Autodesk Inventor part; units mm, degrees
ref_plane "YZ Plane" through (0, 0, 0) normal (1, 0, 0) x (0, 1, 0)
ref_plane "XZ Plane" through (0, 0, 0) normal (0, 1, 0) x (-1, 0, 0)
ref_plane "XY Plane" through (0, 0, 0) normal (0, 0, 1) x (1, 0, 0)
sketch "Sketch1" plane through (0, 0, 0) normal (0, 0, 1) x (1, 0, 0)
  line L0 (-25, -13) -> (25, -13)
  line L1 (25, -13) -> (25, 13)
  line L2 (25, 13) -> (-25, 13)
  line L3 (-25, 13) -> (-25, -13)
  line L4 (-25, -13) -> (25, 13) construction
  line L5 (25, -13) -> (-25, 13) construction
  point P0 (0, 0)
  dimension "d0" = 50
  dimension "d1" = 26
extrude "Extrusion1" add sketch "Sketch1" along normal blind 1.6
sketch "Sketch2" plane through (0, 0, 1.6) normal (0, 0, 1) x (1, 0, 0)
  line L0 (-10.2, -7.5) -> (2.8, -7.5) construction
  line L1 (2.8, -7.5) -> (2.8, 7.5) construction
  line L2 (2.8, 7.5) -> (-10.2, 7.5) construction
  line L3 (-10.2, 7.5) -> (-10.2, -7.5) construction
  line L4 (-25, 13) -> (-25, -13) construction
  point P0 (0, 0)
  point P1 (2.8, 0)
  dimension "d4" = 13
  dimension "d5" = 15
  dimension "d6" = 14.8
hole "Hole1" at (-10.2, 7.5, 1.6) at (2.8, 7.5, 1.6) at (2.8, -7.5, 1.6) at (-10.2, -7.5, 1.6) direction (0, 0, -1) diameter 4.5 end through all
sketch "Sketch3" plane through (25, -13, 0) normal (1, 0, 0) x (0, 0, -1)
  line L0 (0, 10.5) -> (-6.5, 10.5)
  line L1 (-6.5, 10.5) -> (-6.5, 15.5)
  line L2 (-6.5, 15.5) -> (0, 15.5)
  line L3 (0, 15.5) -> (0, 10.5)
  line L4 (0, 0) -> (0, 26)
  point P0 (0, 13)
  point P1 (0, 13)
  point P2 (0, 13)
  point P3 (0, 13)
  dimension "d14" = 5
  dimension "d15" = 6.5
extrude "Extrusion2" add sketch "Sketch3" along normal mid plane 16
properties part number "IGBT_Platine"
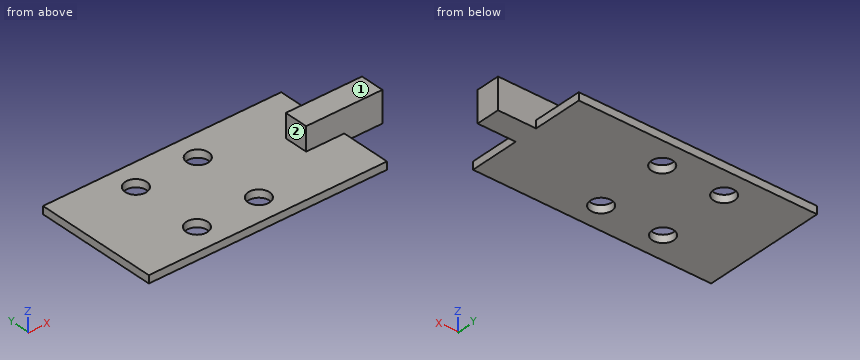
Check sheet for the modelled part. Datum: model origin and axes. Units: mm. Face numbers are marked on the shaded views. A direction names the side the tool comes from. Round coordinates to 2 decimals unless told otherwise and drop trailing zeros. Loops run counter-clockwise (first coordinate to the right, second up) from the corner with the lowest first, then second, coordinate; pieces in that order, holes last. Notation, with made-up numbers: (21.25, 4.25) -> (69.25, 4.25) arc R31 ccw to (69.25, 37.25) -> close; hole circle Ø6 at (-31.5, 4). An arc over 180 degrees is marked (long way). Write item = value, one per line. Start each with the question number.
1) Sectioned sample at C-C, the plane x = 19.5. Record the cut outline in (y, z), plus the area to 3 significant figures.
2) Sectioned sample at B-B, the plane x = -10.2. Record the cut outline in (y, z), plus the area to 3 significant figures.
3) Sectioned sample at D-D, the plane z = 5.25. Record the cut outline in (x, y).
4) Thickness scan on probe 1 along Y at (x, z) = (2.8, 0.55); probe 2 along X at (y, z) = (-7.5, 0.6); probe 3 along Z at (x, y) = (21, -6.25). Record the ranges inside material, lowest first.
5) Gauge pin test, flat ends, axial feed: pin 1 Ø0.8 at (y, z) = (7, 1) entering from +X; pin 2 Ø1 at (x, y) = (-3, 6.5) entering from +Z; pin 3 Ø3 at (y, z) = (2, 4.5) entering from -X; pin 4 Ø4 at (x, y) = (-10.2, 7.5) entering from -Z. Record the tip position at first contact, or that the pin passes through.
6) Set-up check for the marked faces 1 and 2: record each of +Z, -Z, +X, -X, +Y, -Y from which the full face is reachable in a straight line by a thin tool's end or side.
7) Sectioned sample at A-A, the plane y = -7.5. Record the cut outline in (x, z), plus the area to 3 significant figures.
Results are:
q1.outline = (-13, 0) -> (13, 0) -> (13, 1.6) -> (2.5, 1.6) -> (2.5, 6.5) -> (-2.5, 6.5) -> (-2.5, 1.6) -> (-13, 1.6) -> close
q1.area = 66.1 mm^2
q2.outline = (-13, 0) -> (-9.75, 0) -> (-9.75, 1.6) -> (-13, 1.6) -> close; (-5.25, 0) -> (5.25, 0) -> (5.25, 1.6) -> (-5.25, 1.6) -> close; (9.75, 0) -> (13, 0) -> (13, 1.6) -> (9.75, 1.6) -> close
q2.area = 27.2 mm^2
q3.outline = (17, -2.5) -> (33, -2.5) -> (33, 2.5) -> (17, 2.5) -> close
q4.probe_1 = -13 to -9.75, -5.25 to 5.25, 9.75 to 13
q4.probe_2 = -25 to -12.45, -7.95 to 0.55, 5.05 to 25
q4.probe_3 = 0 to 1.6
q5.pin_1 = 25
q5.pin_2 = 1.6
q5.pin_3 = 17
q5.pin_4 = through
q6.face_1 = +Z, +X, -X, +Y, -Y
q6.face_2 = +Z, -X, +Y, -Y
q7.outline = (-25, 0) -> (-12.45, 0) -> (-12.45, 1.6) -> (-25, 1.6) -> close; (-7.95, 0) -> (0.55, 0) -> (0.55, 1.6) -> (-7.95, 1.6) -> close; (5.05, 0) -> (25, 0) -> (25, 1.6) -> (5.05, 1.6) -> close
q7.area = 65.6 mm^2
